Input: part model. Units: mm. Frame: model coordinates. Face numbers are marked on the shaded views. Give positions to 0.01 mm unless a question says otherwise; leave off trailing zeros. Loops run counter-clockwise (first coordinate to the right, second up) from the corner with the lowest first, then second, coordinate; pieces in that order, holes last. Notation, with made-up numbers: M -20,-24 L 37,-24 A31 ccw 37,5 Z; hole C -19.5,-9 d2. An arc over 180 degrees is marked long. Use a Markdown table: item, result. Add a question column.
from build123d import *

# Parameters (mm, degrees)
F1_DEPTH = 30
F2_R     = 3.7
F3_DEPTH = 15


with BuildPart() as f1:
    # F0 (on Top) → F1 (new body)
    with BuildSketch(Plane.XY):
        Polygon((4.943737, 8.692737), (-5.056263, 8.627771), (-10, -0.064966), (-4.943737, -8.692737), (5.056263, -8.627771), (10, 0.064966), align=None)
    extrude(amount=F1_DEPTH)

    # F2 (on face) → F3 (cut)
    with BuildSketch(Plane(origin=(0, 0, 0), x_dir=(1, 0, 0), z_dir=(0, 0, -1))):
        Circle(F2_R)
    extrude(amount=-F3_DEPTH, mode=Mode.SUBTRACT)


solid = f1.part
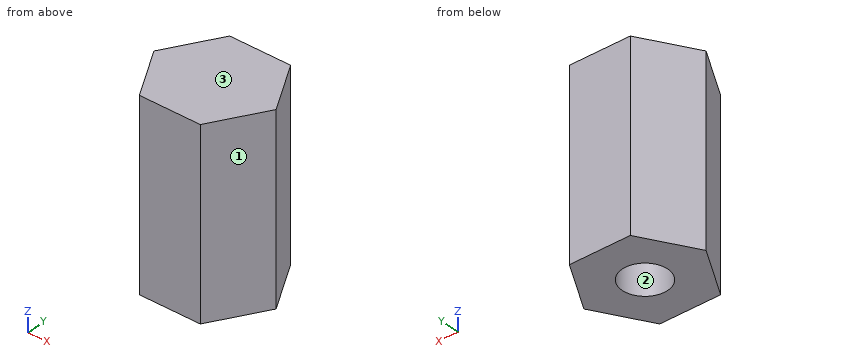
1) Ray query, line 1 (Z direction, x = -0.75, y = 0); line 2 (X direction, y = 0, z = 5.75); line 3 (Y direction, x = 0, z = 10). Return the intervals inside material, ascending. Write a range as [from, to].
2) Section query B-B, the plane y = -0.5. Return the cut outline in (x, z).
3) Section query A-A, the plane z = 22.25. Return the cut outline in (x, y).
4) Section query C-C, the plane x = -2.5. Return the cut outline in (y, z), and give its area (3 significant figures).
5) Contact query for flat-ended pins moving along their axis: P1, Ø8, axis at x = -1.5, z = 11.5, coming from the +Y side; P2, Ø1, axis at y = -7, z = 8.5, coming from the +X side; P3, Ø5, axis at y = 6.5, z = 18, coming from the +X side. Output: stop coordinate, or through.
6) Section query D-D, the plane y = 4.75. Return the cut outline in (x, z).
7) Pull-direction query (Y, two-part tool) for the marked faces 1, 2 and 3; classes: pulls with the +Y half, pulls with the -Y half, needs draft (parallel to the pull), parting line crosses it, or undercut.
Entries:
| question | item | result |
|---|---|---|
| 1 | line 1 | z = [15, 30] |
| 1 | line 2 | x = [-9.96, -3.7], [3.7, 9.96] |
| 1 | line 3 | y = [-8.66, -3.7], [3.7, 8.66] |
| 2 | outline | M -9.75,0 L -3.67,0 L -3.67,15 L 3.67,15 L 3.67,0 L 9.68,0 L 9.68,30 L -9.75,30 Z |
| 3 | outline | M -10,-0.06 L -4.94,-8.69 L 5.06,-8.63 L 10,0.06 L 4.94,8.69 L -5.06,8.63 Z |
| 4 | outline | M -8.68,0 L -2.73,0 L -2.73,15 L 2.73,15 L 2.73,0 L 8.64,0 L 8.64,30 L -8.68,30 Z |
| 4 | area | 438 mm² |
| 5 | P1 | stops at y = 8.68 |
| 5 | P2 | stops at x = 6.27 |
| 5 | P3 | stops at x = 7.69 |
| 6 | outline | M -7.26,0 L 7.25,0 L 7.25,30 L -7.26,30 Z |
| 7 | face 1 | pulls with the -Y half |
| 7 | face 2 | undercut |
| 7 | face 3 | needs draft |
